Can you work these out from the drawing? Everything is in mm from the part's minimum corner. Coordinates: 2 decimals unless noted, no trailing zeros. Loops run counter-clockwise (first coordinate to the right, second up) from the corner with the lowest first, then second, coordinate; pieces in that order, holes last.
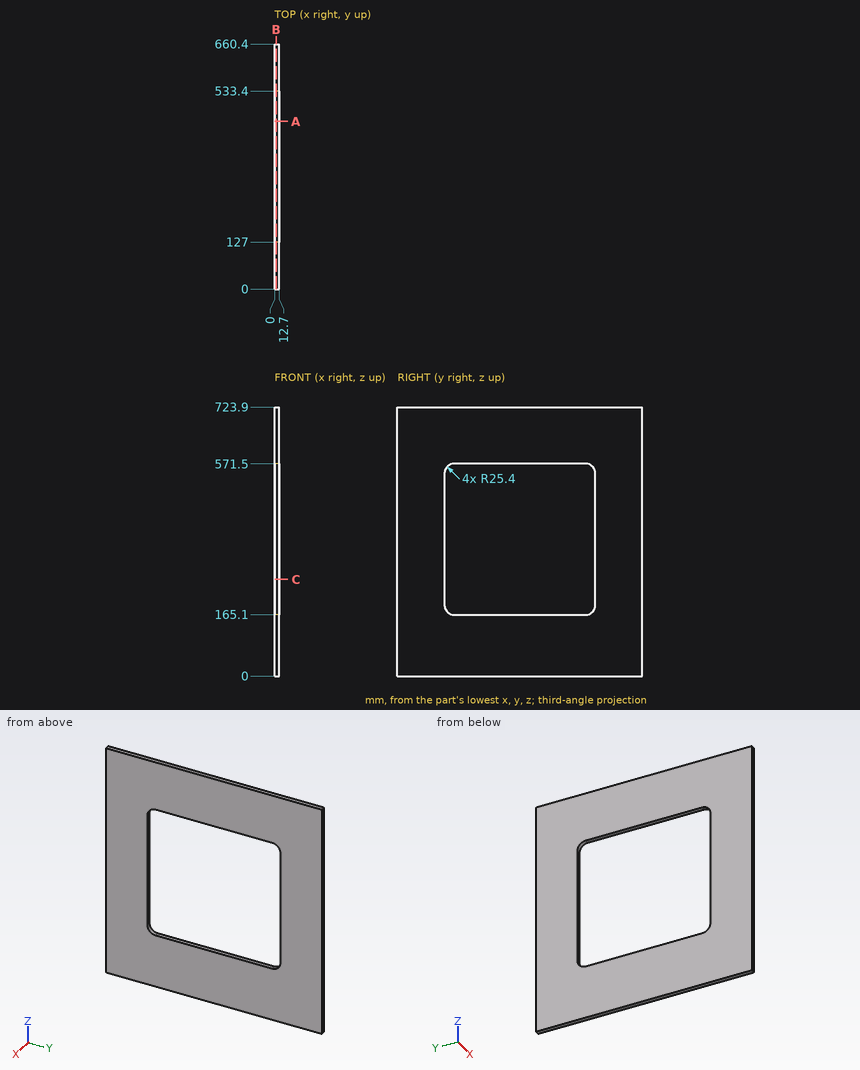
(1) For pin 1 (3 mm diameter, centred on x = 3.5, y = 323.5, fed in from -Z), with a flat end and sliding along its axis, tell me the tip position at first contact or that it passes through.
Answers:
pin 1: stops at z = 0
(2) Imagine slicing it at A-A, the plane y = 452. Write out the boundary of the cut face in (x, z), and give its area (3 significant figures).
Answers:
outline: (0, 0) - (12.7, 0) - (12.7, 165.1) - (0, 165.1) - close; (0, 571.5) - (12.7, 571.5) - (12.7, 723.9) - (0, 723.9) - close
area: 4,030 mm2
(3) Imagine slicing it at B-B, the plane x = 4. Write out the boundary of the cut face in (y, z), and give its area (3 significant figures).
Answers:
outline: (0, 0) - (660.4, 0) - (660.4, 723.9) - (0, 723.9) - close; hole (127, 190.5) arc R25.4 ccw to (152.4, 165.1) - (508, 165.1) arc R25.4 ccw to (533.4, 190.5) - (533.4, 546.1) arc R25.4 ccw to (508, 571.5) - (152.4, 571.5) arc R25.4 ccw to (127, 546.1) - close
area: 313,000 mm2
(4) Imagine slicing it at C-C, the plane z = 260. Write out the boundary of the cut face in (x, y), and give its area (3 significant figures).
Answers:
outline: (0, 0) - (12.7, 0) - (12.7, 127) - (0, 127) - close; (0, 533.4) - (12.7, 533.4) - (12.7, 660.4) - (0, 660.4) - close
area: 3,230 mm2
(5) I need wall thicknesses on probe 1 along Y at (x, z) = (8.75, 193.5); probe 2 along Z at (x, y) = (7.5, 374.5). Which ranges of each line are inside material? Lowest first, please.
Answers:
probe 1: y = 0 to 127, 533.4 to 660.4
probe 2: z = 0 to 165.1, 571.5 to 723.9
